Read the model definition and answer for the solid it produces. Units are mm, in the model's axes. A direction names the side the tool comes from. Round coordinates to 2 decimals unless told otherwise and drop trailing zeros. Order: outer loops, then holes, each group sorted by start corner. A loop starts at its lowest first (then second) coordinate and runs counter-clockwise, first axis right, second up.
from build123d import *

# Parameters (mm, degrees)
F0_W          = 5.842
F0_H          = 12.7
F0_R          = 3.175
F2_DEPTH      = 3.175
F3_R          = 1.524
F4_DEPTH      = 6.35
F4_DEPTH_BACK = 1.27
F5_R          = 1.524
F6_DEPTH      = 10.414
F7_R          = 1.524
F8_DEPTH      = 17.78
F9_DEPTH      = 56.134
F10_R         = 1.27
F11_T1_DEPTH  = 27.94
F11_T4_ANGLE  = 180


# Not quite as in the source:
# - a fillet or chamfer that OpenCascade refuses, or shapes differently, is made with other operations: its cross-section is extruded or revolved along the edge and cut away or added


with BuildPart() as f1:
    # F0 (on Front) → F1 (revolve)
    with BuildSketch(Plane.XZ):
        Polygon((5.842, 12.7), (5.842, 0), (66.294, 0), (66.294, 12.7), (56.134, 12.7), (56.134, 10.16), (10.16, 10.16), (10.16, 12.7), align=None)
        with Locations((2.921, 6.35)):
            Rectangle(F0_W, F0_H)
    revolve(axis=Axis((33.147, 0, 0), (-1, 0, 0)))

    # F0 (on Front) → F2 (join, symmetric)
    with BuildSketch(Plane.XZ):
        with BuildLine():
            Line((-0.9398, 0), (0, 0))
            Line((0, 0), (0, 12.7))
            Line((0, 12.7), (5.842, 12.7))
            Line((5.842, 12.7), (5.842, 15.24))
            Line((5.842, 15.24), (-0.508, 15.24))
            Line((-0.508, 15.24), (-10.8806298187, 3.8475430269))
            ThreePointArc((-10.8806298187, 3.8475430269), (-4.5919612295, 5.3297205562), (-0.9398, 0))
        make_face()
        with Locations((2.921, 6.35)):
            Rectangle(F0_W, F0_H)
        with BuildLine():
            Line((5.842, 0), (0, 0))
            Line((0, 0), (-0.9398, 0))
            ThreePointArc((-0.9398, 0), (-3.1957909266, -4.5493385486), (-8.1826630726, -5.5069827884))
            Line((-8.1826630726, -5.5069827884), (5.842, -9.398))
            Line((5.842, -9.398), (5.842, 0))
        make_face()
        with BuildLine():
            ThreePointArc((-8.1826630726, -5.5069827884), (-3.1957909266, -4.5493385486), (-0.9398, 0))
            ThreePointArc((-0.9398, 0), (-4.5919612295, 5.3297205562), (-10.8806298187, 3.8475430269))
            ThreePointArc((-10.8806298187, 3.8475430269), (-12.1459778134, -1.5837270034), (-8.1826630726, -5.5069827884))
        make_face()
        with Locations((-6.6548, 0)):
            Circle(F0_R, mode=Mode.SUBTRACT)
    extrude(amount=F2_DEPTH, both=True)

    # F3 (on face) → F4 (join, two sides)
    with BuildSketch(Plane.YZ.offset(66.294)) as f4_sk:
        with BuildLine():
            ThreePointArc((-5.08, 0), (0, -5.08), (5.08, 0))
            ThreePointArc((5.08, 0), (0, 5.08), (-5.08, 0))
        make_face()
        Circle(F3_R, mode=Mode.SUBTRACT)
        with BuildLine():
            ThreePointArc((-5.08, 0), (0, 5.08), (5.08, 0))
            Line((5.08, 0), (5.08, 15.24))
            Line((5.08, 15.24), (-5.08, 15.24))
            Line((-5.08, 15.24), (-5.08, 0))
        make_face()
    extrude(amount=F4_DEPTH)
    extrude(f4_sk.sketch, amount=-F4_DEPTH_BACK)

    # F5 (on face) → F6 (cut)
    with BuildSketch(Plane.XY.offset(15.24)):
        with Locations((68.834, 0)):
            Circle(F5_R)
    extrude(amount=-F6_DEPTH, mode=Mode.SUBTRACT)

    # F7 (on face) → F8 (cut)
    with BuildSketch(Plane.XY.offset(15.24)):
        with Locations((2.667, 0)):
            Circle(F7_R)
    extrude(amount=-F8_DEPTH, mode=Mode.SUBTRACT)

    # F9 (cut, through all): a face of the model
    f9_faces = [f1.faces().sort_by_distance(p)[0] for p in [
        (66.294, 0, 0),
    ]]
    extrude(f9_faces, amount=-F9_DEPTH, mode=Mode.SUBTRACT)

    # F10
    f10_edges = [f1.edges().sort_by_distance(p)[0] for p in [
        (-12.145978, 3.175, -1.583727),
        (-5.694315, 3.175, 9.543772),
    ]]
    fillet(f10_edges, radius=F10_R)

    # F11: fillet of radius 5.08 on 2 edges, made by hand

    # F11_s2 → F11_t1 (cut)
    with BuildSketch(Plane.XY):
        with BuildLine():
            ThreePointArc((67.564, -5.08), (71.1561024484, -3.5921024484), (72.644, 0))
            Line((72.644, 0), (72.644, -5.08))
            Line((72.644, -5.08), (67.564, -5.08))
        make_face()
        with BuildLine():
            ThreePointArc((67.564, 5.08), (71.1561024484, 3.5921024484), (72.644, 0))
            Line((72.644, 0), (72.644, 5.08))
            Line((72.644, 5.08), (67.564, 5.08))
        make_face()
    extrude(amount=F11_T1_DEPTH, mode=Mode.SUBTRACT)

    # F11_s3 → F11_t4 (revolve, cut)
    with BuildSketch(Plane.XY):
        with BuildLine():
            ThreePointArc((67.564, -5.08), (71.1561024484, -3.5921024484), (72.644, 0))
            Line((72.644, 0), (72.644, -5.08))
            Line((72.644, -5.08), (67.564, -5.08))
        make_face()
    revolve(axis=Axis((72.644, 0, 0), (1, 0, 0)), revolution_arc=F11_T4_ANGLE, mode=Mode.SUBTRACT)


solid = f1.part
Q1. Straight lines are drawn through the part: probe 1 along Z at (x, y) = (59, 0); probe 2 along X at (y, z) = (8.5, -4); probe 3 along Y at (x, z) = (14.5, -0.75). For each, find the intervals that lie inside material, in ascending order.
Outcome:
probe 1: z = -12.7 to -1.52, 1.52 to 12.7
probe 2: x = 0 to 66.29
probe 3: y = -10.13 to -1.33, 1.33 to 10.13
Q2. A cutting plane is placed at D-D, the plane z = 13.5. Give the number of separate pieces and of enclosed holes in the cut face, plus the area to 3 significant figures.
Outcome:
separate pieces: 2
enclosed holes: 2
area: 102 mm2
Q3. For a pull along Y with two mould halves and no side action, classify faces 6 (the face through (10.16, 0, 0)), 7 (the face through (5.01, -12.4, -2.75)), 8 (the face through (65.024, 0, 14)), 9 (the face through (70.288, 0.458, 10.106)) as released by +Y, released by -Y, zero draft, split by the parting line, or undercut.
Outcome:
face 6: undercut
face 7: split by the parting line
face 8: zero draft
face 9: undercut
Q4. For faces 1 (the face through (32.825, 10.074, -1.323)), 2 (the face through (66.294, 0, -6)), 3 (the face through (67, -5.08, 9)), 4 (the face through (67, 5.08, 9)), 5 (the face through (4.12, 0.46, 6.47)), determine the directions among +Z, -Z, +X, -X, +Y, -Y from which every point of the face is accessible in a straight line to the end or side of a thin tool.
Outcome:
face 1: none
face 2: -Z, +X
face 3: +Z, +X, -Y
face 4: +Z, +X, +Y
face 5: +Z
Q5. Flat-ended cylindrical pins translate along their axes: pin 1 (2 mm diameter, centred on x = 32, z = 4, fed in from +Y); pin 2 (6 mm diameter, centred on x = 32.5, y = -5, fed in from +Z); pin 3 (12 mm diameter, centred on y = -6.5, z = -4.5, fed in from -X); pin 4 (13.5 mm diameter, centred on x = -2.5, z = 7, fed in from +Y). Find the tip coordinate at first contact, or state that the pin passes through.
Outcome:
pin 1: stops at y = 9.71
pin 2: stops at z = 9.96
pin 3: stops at x = -12.37
pin 4: stops at y = 12.68
Q6. A cutting plane is placed at A-A, the plane y = -9.25. Give the vertices of the cut face in (x, z), plus the area to 3 significant figures.
Outcome:
outline: (0, -8.7) - (10.16, -8.7) - (10.16, -4.2) - (56.13, -4.2) - (56.13, -8.7) - (66.29, -8.7) - (66.29, 8.7) - (56.13, 8.7) - (56.13, 4.2) - (10.16, 4.2) - (10.16, 8.7) - (0, 8.7) - close
area: 740 mm2
Q7. A cutting plane is placed at B-B, the plane x = 19.5. Give the vertices of the cut face in (y, z).
Outcome:
outline: circle Ø20.32 at (0, 0); hole circle Ø3.05 at (0, 0)
